Design review of the part shown in the three views and the two pictorial views. Dimensions are in mm from the part's minimum x, y and z. A direction names the side the tool comes from. Give positions to 0.01 mm unless a question says otherwise; leave off trailing zeros. Order: outer loops, then holes, each group sorted by start corner. A loop starts at its lowest first (then second) coordinate and runs counter-clockwise, first axis right, second up. Notation, with made-up numbers: M 52.5,-12.75 L 76.5,-12.75 A27 ccw 76.5,9.25 Z; hole C 5,-15.75 d7. An arc over 180 degrees is marked long. Answer as a JSON object with one key per item and string values.
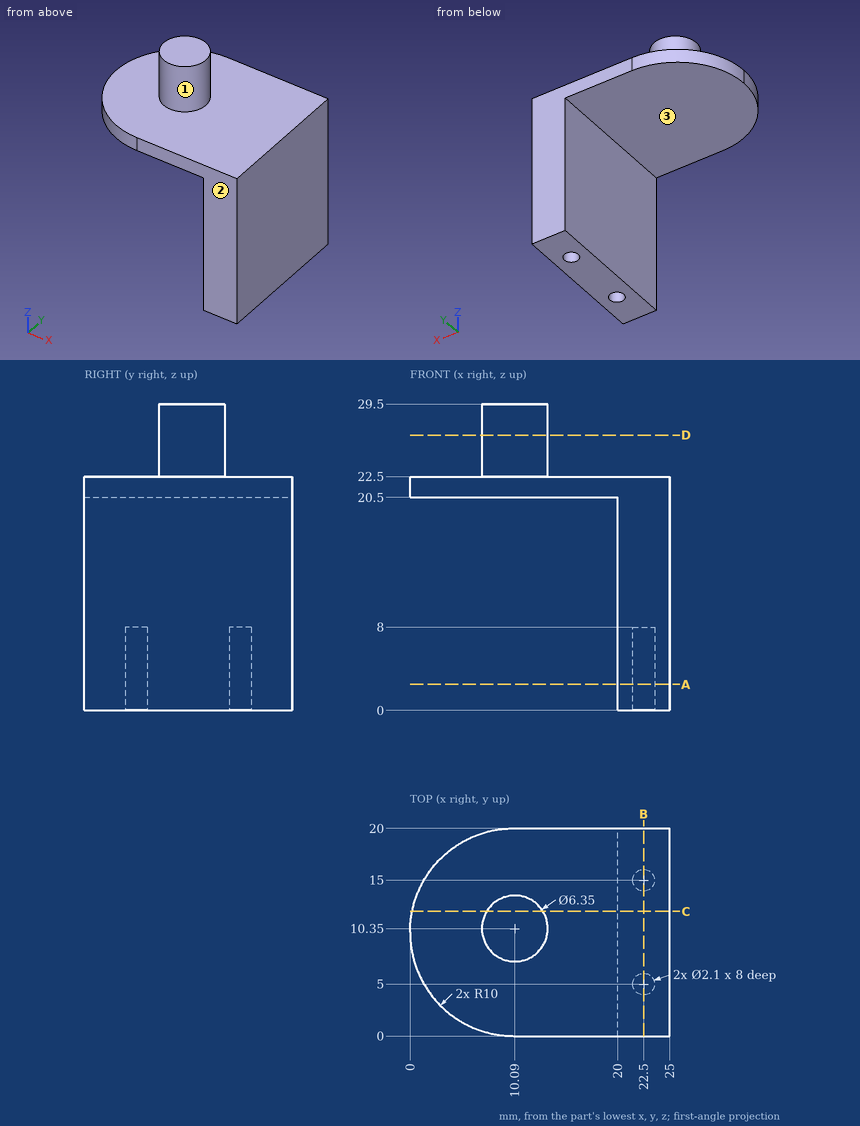
(1) To check wall thickness, follow L1, parallel to Y at x = 22.5, z = 2; L2, parallel to Z at x = 2.25, y = 15; L3, parallel to Z at x = 22.5, y = 17.5. State the ranges of each line that lie inside material, in increasing order. Write a range as from..to.
Checked values:
{"L1": "y = 0..3.95, 6.05..13.95, 16.05..20", "L2": "z = 20.5..22.5", "L3": "z = 0..22.5"}
(2) We need section A-A (z = 2.5). Write out the cut boundary in (x, y), plus the area to 3 significant figures.
Checked values:
{"outline": "M 20,0 L 25,0 L 25,20 L 20,20 Z; hole C 22.5,5 d2.1; hole C 22.5,15 d2.1", "area": "93.1 mm^2"}
(3) Tool access review of the marked faces 1, 2 and 3: name each direction out of +Z, -Z, +X, -X, +Y, -Y from which nothing blocks a thin tool from reaching the whole face with its end or side.
Checked values:
{"face 1": "+Z", "face 2": "+Z, -Z, +X, -X, -Y", "face 3": "-Z, -X, +Y, -Y"}
(4) We need section B-B (x = 22.5). Write out the cut boundary in (y, z), plus the area to 3 significant figures.
Checked values:
{"outline": "M 0,0 L 3.95,0 L 3.95,8 L 6.05,8 L 6.05,0 L 13.95,0 L 13.95,8 L 16.05,8 L 16.05,0 L 20,0 L 20,22.5 L 0,22.5 Z", "area": "416 mm^2"}
(5) Insertion check: pin 1 (1.3 mm diameter, centred on x = 22.5, y = 15, fed in from +Z); pin 2 (10 mm diameter, centred on x = 11, y = 6, fed in from -Z); pin 3 (12 mm diameter, centred on y = 6.5, z = 11, fed in from -X). Each pin has a flat end and moves straight along its axis. Give the tip position at first contact, or say it passes through.
Checked values:
{"pin 1": "stops at z = 22.5", "pin 2": "stops at z = 20.5", "pin 3": "stops at x = 20"}
(6) We need section C-C (y = 12). Write out the cut boundary in (x, z).
Checked values:
{"outline": "M 0.2,20.5 L 20,20.5 L 20,0 L 25,0 L 25,22.5 L 12.8,22.5 L 12.8,29.5 L 7.38,29.5 L 7.38,22.5 L 0.2,22.5 Z"}
(7) We need section D-D (z = 26.5). Write out the cut boundary in (x, y) (3 decimals).
Checked values:
{"outline": "C 10.09,10.35 d6.35"}
